Solid Edge part; units mm, degrees
sketch "Sketch1" plane through (0, 0, 0) normal (0, 0, 1) x (1, 0, 0)
  circle A0 centre (0, 0) radius 41.05
  circle A1 centre (0, 0) radius 20.625
  circle A2 centre (164.42, 0) radius 23.37
  circle A3 centre (164.42, 0) radius 13.21
extrude "Protrusion1" add sketch "Sketch1" along normal blind 17.73
sketch "Sketch2" plane through (0, 0, 0) normal (0, 0, 1) x (1, 0, 0)
  line L0 (164.42, -23.37) -> (8.6399, -40.1305)
  line L1 (31.0664, 0) -> (8.6399, -40.1305)
  line L2 (8.6399, 40.1305) -> (31.0664, 0)
  line L3 (164.42, 23.37) -> (8.6399, 40.1305)
  line L4 (143.9301, 0) -> (164.42, 23.37)
  line L5 (164.42, -23.37) -> (143.9301, 0)
extrude "ExtrudedProtrusion_2" add sketch "Sketch2" along normal blind 12.7
sketch "Sketch3" plane through (0, 0, 0) normal (0, 0, 1) x (1, 0, 0)
  line L0 (-5.0968, -15.4278) -> (-7.5968, -19.758)
  line L1 (-13.3125, -16.458) -> (-7.5968, -19.758)
  line L2 (-10.8125, -12.1278) -> (-13.3125, -16.458)
  line L3 (-5.0968, -15.4278) -> (-10.8125, -12.1278)
  line L4 (-10.8125, 12.1278) -> (-5.0968, 15.4278)
  line L5 (-5.0968, 15.4278) -> (-7.5968, 19.758)
  line L6 (-7.5968, 19.758) -> (-13.3125, 16.458)
  line L7 (-10.8125, 12.1278) -> (-13.3125, 16.458)
  line L8 (15.9093, -3.3) -> (20.9093, -3.3)
  line L9 (20.9093, -3.3) -> (20.9093, 3.3)
  line L10 (15.9093, 3.3) -> (20.9093, 3.3)
  line L11 (15.9093, 3.3) -> (15.9093, -3.3)
extrude "Protrusion2" add sketch "Sketch3" along normal up to vertex (17.73 mm away)
Can you work these out from the model? Positions are in its coordinate system, mm. A direction names the side the tool comes from. Coordinates: 2 decimals unless noted, no trailing zeros. Loops run counter-clockwise (first coordinate to the right, second up) from the corner with the lowest first, then second, coordinate; pieces in that order, holes last. Notation, with made-up numbers: (33, -26.5) - (78, -26.5) arc R13 cw to (78, -15.5) - close; hole circle Ø10 at (-1, 63). An arc over 180 degrees is marked (long way). Put each result on its own line as item: value. Start each with the question number.
Item 1: Suppose I cut it at C-C (x = 0). Please give me the cut outline in (y, z) (3 decimals).
Item 2: Which directions (+Z, -Z, +X, -X, +Y, -Y) give clear straight access to the entire face, cutting with the end or side of a thin tool? Please do faces 5 (the face through (-6.194, -17.328, 8.741)), 6 (the face through (18, 1, 17.73)), 7 (the face through (186.71, -7.02, 10.71)).
Item 3: Suppose I cut it at A-A (y = 0). Please give me the cut outline in (x, z) (3 decimals).
Item 4: Suppose I cut it at D-D (x = 147). Please give me the cut outline in (y, z), and give its area (3 significant figures).
Item 5: If we mould it in two halves opening along Y, with no side actions, what happens to faces 1 (the face through (88, 1, 12.7)), 2 (the face through (-11.91, 14.03, 8.74)), 3 (the face through (10.533, -17.732, 8.741)), 4 (the face through (87.62, -31.633, 6.261))? For each: +Y half, -Y half, draft (parallel to the pull), parting line (faces both ways), or undercut.
Item 6: If I drill on line 1 along Y through (x, z) = (164.42, 4.75); line 2 along Y through (x, z) = (-6.5, 4.5); line 3 along X through (y, z) = (-11, 13), over which ranges is the centre line in solid material (lowest first)?
Item 7: Suppose I cut it at B-B (z = 10.5). State how many separate pieces and enclosed holes the cut face has, and give its area (3 significant figures).
Item 8: For pin 1 (24 mm diameter, centred on x = 124, y = 1.5, fed in from +Z); pin 2 (5 mm diameter, centred on x = 142, z = 10, fed in from +Y); pin 3 (3 mm diameter, centred on x = 1, z = 15, fed in from +Y), each with a flat end and sliding along its axis, tell me the tip position at first contact or that it passes through.
Here are the results:
1. outline: (-41.05, 0) - (-20.625, 0) - (-20.625, 17.73) - (-41.05, 17.73) - close; (20.625, 0) - (41.05, 0) - (41.05, 17.73) - (20.625, 17.73) - close
2. face 5: +Z, -Z
2. face 6: +Z, +X, -X, +Y, -Y
2. face 7: +Z
3. outline: (-41.05, 0) - (-20.625, 0) - (-20.625, 17.73) - (-41.05, 17.73) - close; (15.909, 0) - (151.21, 0) - (151.21, 17.73) - (141.05, 17.73) - (141.05, 12.7) - (41.05, 12.7) - (41.05, 17.73) - (15.909, 17.73) - close; (177.63, 0) - (187.79, 0) - (187.79, 17.73) - (177.63, 17.73) - close
4. outline: (-25.24, 0) - (25.24, 0) - (25.24, 12.7) - (15.58, 12.7) - (15.58, 17.73) - (-15.58, 17.73) - (-15.58, 12.7) - (-25.24, 12.7) - close
4. area: 798 mm²
5. face 1: draft
5. face 2: undercut
5. face 3: undercut
5. face 4: -Y half
6. line 1: -23.37 to -13.21, 13.21 to 23.37
6. line 2: -40.53 to -19.57, -17.86 to -14.62, 14.62 to 17.86, 19.57 to 40.53
6. line 3: -39.55 to -17.45, 17.45 to 39.55, 143.8 to 157.11, 171.73 to 185.04
7. separate pieces: 1
7. enclosed holes: 2
7. area: 12,300 mm²
8. pin 1: z = 12.7
8. pin 2: y = 26.05
8. pin 3: y = 41.05
